Answer from the drawing. Dimensions are ordinates in mm from the lowest x, y and z of the part. Give positions to 0.01 mm unless a question says otherwise; leave off trailing zeros. Loops run counter-clockwise (first coordinate to the right, second up) from the corner with the lowest first, then second, coordinate; pieces in that order, holes last. Notation, with made-up numbers: (-35.5, -21.5) - (17.5, -21.5) arc R9 cw to (17.5, -13.5) - close; hole circle Ø11 at (-18.75, 86). An arc over 180 degrees is marked (long way). Write each question's results on one line, items separated by ' | '. Start each with the question number.
Q1. The part is cut by section A-A, the plane y = 6. Write down the section's boundary in (x, z).
Q2. Find the intervals of material crossed by line 1 (Y direction, x = 4, z = 0.9); line 2 (Y direction, x = 37.5, z = 0.5); line 3 (X direction, y = 25.5, z = 0.3), in increasing order. Write a range as from..to.
Q3. Given pin 1 (4.5 mm diameter, centred on x = 4.25, y = 18.25, fed in from +Z); pin 2 (8 mm diameter, centred on x = 45.5, y = 22, fed in from +Z), each flat-ended and moving along its own axis, determine where each tip first touches the part or whether it passes through.
Q4. The part is cut by section C-C, the plane z = 0.85. State how many separate pieces and enclosed holes the cut face has.
Q5. The part is cut by section D-D, the plane y = 18.25. Write down the section's boundary in (x, z) (1 decimal).
Q6. The part is cut by section B-B, the plane x = 14.5. Write down the section's boundary in (y, z).
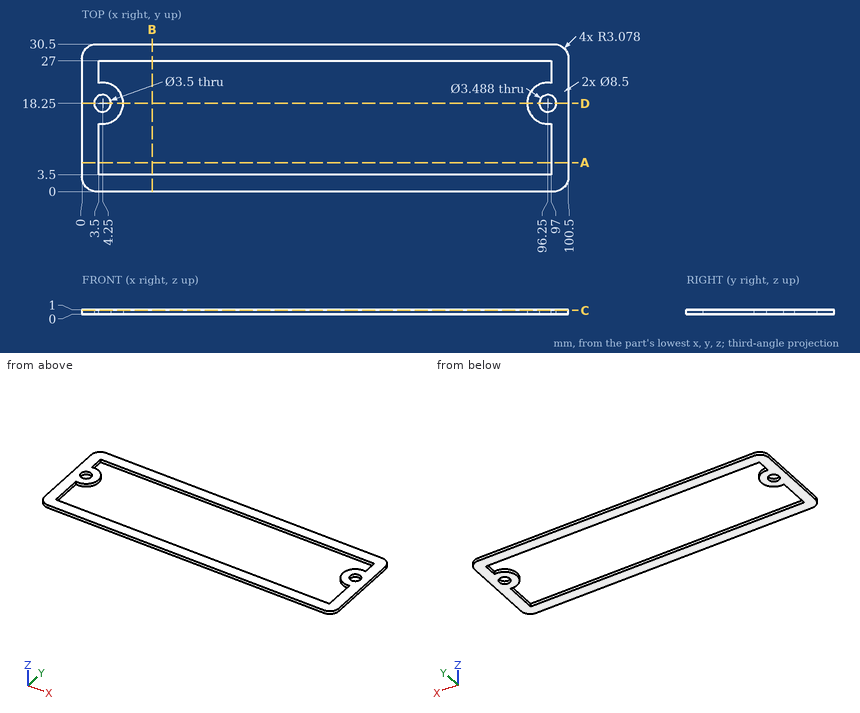
Check sheet entries:
1) outline: (0, 0) - (3.5, 0) - (3.5, 1) - (0, 1) - close; (97, 0) - (100.5, 0) - (100.5, 1) - (97, 1) - close
2) line 1: y = 0..3.5, 14.01..16.52, 19.98..22.49, 27..30.5 | line 2: y = 0..3.5, 27..30.5 | line 3: x = 0..3.5, 97..100.5
3) pin 1: stops at z = 1 | pin 2: passes through
4) separate pieces: 1 | enclosed holes: 3
5) outline: (0, 0) - (2.5, 0) - (2.5, 1) - (0, 1) - close; (6, 0) - (8.5, 0) - (8.5, 1) - (6, 1) - close; (92, 0) - (94.5, 0) - (94.5, 1) - (92, 1) - close; (98, 0) - (100.5, 0) - (100.5, 1) - (98, 1) - close
6) outline: (0, 0) - (3.5, 0) - (3.5, 1) - (0, 1) - close; (27, 0) - (30.5, 0) - (30.5, 1) - (27, 1) - close
